Autodesk Inventor part; units mm, degrees
ref_plane "YZ Plane" through (0, 0, 0) normal (1, 0, 0) x (0, 1, 0)
ref_plane "XZ Plane" through (0, 0, 0) normal (0, 1, 0) x (-1, 0, 0)
ref_plane "XY Plane" through (0, 0, 0) normal (0, 0, 1) x (1, 0, 0)
sketch "Sketch1" plane through (0, 0, 0) normal (0, 1, 0) x (-1, 0, 0)
  circle A0 centre (0, 0) radius 9.75
  circle A1 centre (0, 0) radius 11.75
  dimension "d0" = 19.5
  dimension "d1" = 23.5
extrude "Extrusion1" add sketch "Sketch1" along normal blind 2 contours A0 | A1
sketch "Sketch2" plane through (0, 2, 0) normal (0, 1, 0) x (1, 0, 0)
  circle A0 centre (0, 0) radius 9.75
  dimension "d4" = 19.5
extrude "Extrusion2" cut sketch "Sketch2" against normal blind 1
sketch "Sketch3" plane through (0, 1, 0) normal (0, 1, 0) x (1, 0, 0)
  circle A0 centre (0, 0) radius 8.75
  dimension "d7" = 17.5
extrude "Extrusion3" cut sketch "Sketch3" against normal blind 1
sketch "Sketch4" plane through (0, 0, 0) normal (0, -1, 0) x (1, 0, 0)
  circle A0 centre (0, 0) radius 8.75
  circle A1 centre (0, 0) radius 10.75
  dimension "d10" = 21.5
  dimension "d13" = 17.5
extrude "Extrusion4" add sketch "Sketch4" along normal blind 6
properties part number "685ZZFlanged_Adapter_4mm"
Can you work these out from the model? Positions are in its coordinate system, mm. A direction names the side the tool comes from. Coordinates: 2 decimals unless noted, no trailing zeros. Write each loop counter-clockwise with the first axis right and the second up, starting at its lowest first coordinate (ties: lowest second). Pieces come first, ordered by that corner, then holes. Notation, with made-up numbers: (77, 75) -> (136, 75) arc R28 cw to (136, 104) -> close; hole circle Ø7 at (12, 80). An arc over 180 degrees is marked (long way). Write each question's results on one line, items separated by ' | '. Start each with the question number.
Q1. I'm going to push flat-ended pins straight in: pin 1 (2 mm diameter, centred on x = 6, z = -2, fed in from -Y); pin 2 (2 mm diameter, centred on y = -5, z = 7.5, fed in from +X). Where does each tip first touch, or does it pass through?
Q2. If I drill on probe 1 along Z at (x, y) = (0, -2.75); probe 2 along Z at (x, y) = (0, 1.4); probe 3 along Y at (x, z) = (10.5, -2.5), over which ranges is the centre line in solid material (lowest first)?
Q3. On a 3-axis mill with a long thin cutter (end or side, diameter ignored), from which of +Z, -Z, +X, -X, +Y, -Y can I reach the whole of each face in a straight line? I mean faces 1 (the face through (-5, 0, -10)), 2 (the face through (-1.269, 1.507, -9.667)), 3 (the face through (2, -6, -9)). Say none if no direction works.
Q4. Imagine slicing it at B-B (z = 0). Write out the boundary of the cut face in (x, y), then the cut area to 3 significant figures.
Q5. Imagine slicing it at A-A (x = 0). Write out the boundary of the cut face in (y, z).
Q6. We'd pull the mould along Z, two halves only. Please class faces 4 (the face through (-8, 1, -4)), 5 (the face through (-11.207, 0.986, -3.529)), 6 (the face through (-2, 2, 10)): +Z half, -Z half, draft (parallel to the pull), parting line (faces both ways), or undercut.
Q7. Imagine slicing it at D-D (x = -9.25). Write out the boundary of the cut face in (y, z), then the cut area to 3 significant figures.
Q8. Imagine slicing it at C-C (y = -1). Write out the boundary of the cut face in (x, z), then the cut area to 3 significant figures.
Taken from the geometry:
1) pin 1: passes through | pin 2: stops at x = 8.56
2) probe 1: z = -10.75 to -8.75, 8.75 to 10.75 | probe 2: z = -11.75 to -9.75, 9.75 to 11.75 | probe 3: y = 0 to 2
3) face 1: -Y | face 2: +Y | face 3: +Z, -Z, +X, -X, -Y
4) outline: (-11.75, 0) -> (-10.75, 0) -> (-10.75, -6) -> (-8.75, -6) -> (-8.75, 1) -> (-9.75, 1) -> (-9.75, 2) -> (-11.75, 2) -> close; (8.75, -6) -> (10.75, -6) -> (10.75, 0) -> (11.75, 0) -> (11.75, 2) -> (9.75, 2) -> (9.75, 1) -> (8.75, 1) -> close | area: 34.0 mm^2
5) outline: (-6, -10.75) -> (0, -10.75) -> (0, -11.75) -> (2, -11.75) -> (2, -9.75) -> (1, -9.75) -> (1, -8.75) -> (-6, -8.75) -> close; (-6, 8.75) -> (1, 8.75) -> (1, 9.75) -> (2, 9.75) -> (2, 11.75) -> (0, 11.75) -> (0, 10.75) -> (-6, 10.75) -> close
6) face 4: undercut | face 5: parting line | face 6: draft
7) outline: (-6, -5.48) -> (0, -5.48) -> (0, -7.25) -> (2, -7.25) -> (2, -3.08) -> (1, -3.08) -> (1, 3.08) -> (2, 3.08) -> (2, 7.25) -> (0, 7.25) -> (0, 5.48) -> (-6, 5.48) -> close | area: 88.5 mm^2
8) outline: circle Ø21.5 at (0, 0); hole circle Ø17.5 at (0, 0) | area: 123 mm^2
